from build123d import *

# Parameters (mm, degrees)
DODANIE_WYCI_GNI_CIE1_DEPTH = 6
WYTNIJ_WYCI_GNI_CIE2_DEPTH  = 4
WYTNIJ_WYCI_GNI_CIE3_DEPTH  = 2


with BuildPart() as part:
    # Szkic1 → Dodanie-wyciągnięcie1 (new body)
    with BuildSketch(Plane.XY):
        with BuildLine():
            Line((-16.5, 21.5), (16.5, 21.5))
            ThreePointArc((16.5, 21.5), (20.035533906, 20.035533906), (21.5, 16.5))
            Line((21.5, 16.5), (21.5, -16.5))
            ThreePointArc((21.5, -16.5), (20.035533906, -20.035533906), (16.5, -21.5))
            Line((16.5, -21.5), (-16.5, -21.5))
            ThreePointArc((-16.5, -21.5), (-20.035533906, -20.035533906), (-21.5, -16.5))
            Line((-21.5, -16.5), (-21.5, 16.5))
            ThreePointArc((-21.5, 16.5), (-20.035533906, 20.035533906), (-16.5, 21.5))
        make_face()
    extrude(amount=DODANIE_WYCI_GNI_CIE1_DEPTH)

    # Szkic2 → Wytnij-wyciągnięcie2 (cut)
    with BuildSketch(Plane.XY.offset(6)):
        with BuildLine():
            Line((-16.5, 1.360589702), (-16.5, -1.360589702))
            ThreePointArc((-16.5, -1.360589702), (-16.720373698, -2.828640251), (-17.362068966, -4.167282908))
            ThreePointArc((-17.362068966, -4.167282908), (-16.217514421, -16.217514421), (-4.167282908, -17.362068966))
            ThreePointArc((-4.167282908, -17.362068966), (-2.828640251, -16.720373698), (-1.360589702, -16.5))
            Line((-1.360589702, -16.5), (1.360589702, -16.5))
            ThreePointArc((1.360589702, -16.5), (2.828640251, -16.720373698), (4.167282908, -17.362068966))
            ThreePointArc((4.167282908, -17.362068966), (16.217514421, -16.217514421), (17.362068966, -4.167282908))
            ThreePointArc((17.362068966, -4.167282908), (16.720373698, -2.828640251), (16.5, -1.360589702))
            Line((16.5, -1.360589702), (16.5, 1.360589702))
            ThreePointArc((16.5, 1.360589702), (16.720373698, 2.828640251), (17.362068966, 4.167282908))
            ThreePointArc((17.362068966, 4.167282908), (16.217514421, 16.217514421), (4.167282908, 17.362068966))
            ThreePointArc((4.167282908, 17.362068966), (2.828640251, 16.720373698), (1.360589702, 16.5))
            Line((1.360589702, 16.5), (-1.360589702, 16.5))
            ThreePointArc((-1.360589702, 16.5), (-2.828640251, 16.720373698), (-4.167282908, 17.362068966))
            ThreePointArc((-4.167282908, 17.362068966), (-16.217514421, 16.217514421), (-17.362068966, 4.167282908))
            ThreePointArc((-17.362068966, 4.167282908), (-16.720373698, 2.828640251), (-16.5, 1.360589702))
        make_face()
    extrude(amount=-WYTNIJ_WYCI_GNI_CIE2_DEPTH, mode=Mode.SUBTRACT)

    # Szkic3 → Wytnij-wyciągnięcie3 (cut)
    with BuildSketch(Plane.XY.offset(2)):
        with BuildLine():
            Line((6.5, -5.5), (12.5, -5.5))
            ThreePointArc((12.5, -5.5), (13.207106781, -5.792893219), (13.5, -6.5))
            Line((13.5, -6.5), (13.5, -12.5))
            ThreePointArc((13.5, -12.5), (13.207106781, -13.207106781), (12.5, -13.5))
            Line((12.5, -13.5), (6.5, -13.5))
            ThreePointArc((6.5, -13.5), (5.792893219, -13.207106781), (5.5, -12.5))
            Line((5.5, -12.5), (5.5, -6.5))
            ThreePointArc((5.5, -6.5), (5.792893219, -5.792893219), (6.5, -5.5))
        make_face()
        with BuildLine():
            Line((6.5, 13.5), (12.5, 13.5))
            ThreePointArc((12.5, 13.5), (13.207106781, 13.207106781), (13.5, 12.5))
            Line((13.5, 12.5), (13.5, 6.5))
            ThreePointArc((13.5, 6.5), (13.207106781, 5.792893219), (12.5, 5.5))
            Line((12.5, 5.5), (6.5, 5.5))
            ThreePointArc((6.5, 5.5), (5.792893219, 5.792893219), (5.5, 6.5))
            Line((5.5, 6.5), (5.5, 12.5))
            ThreePointArc((5.5, 12.5), (5.792893219, 13.207106781), (6.5, 13.5))
        make_face()
        with BuildLine():
            Line((-12.5, -5.5), (-6.5, -5.5))
            ThreePointArc((-6.5, -5.5), (-5.792893219, -5.792893219), (-5.5, -6.5))
            Line((-5.5, -6.5), (-5.5, -12.5))
            ThreePointArc((-5.5, -12.5), (-5.792893219, -13.207106781), (-6.5, -13.5))
            Line((-6.5, -13.5), (-12.5, -13.5))
            ThreePointArc((-12.5, -13.5), (-13.207106781, -13.207106781), (-13.5, -12.5))
            Line((-13.5, -12.5), (-13.5, -6.5))
            ThreePointArc((-13.5, -6.5), (-13.207106781, -5.792893219), (-12.5, -5.5))
        make_face()
        with BuildLine():
            Line((-12.5, 13.5), (-6.5, 13.5))
            ThreePointArc((-6.5, 13.5), (-5.792893219, 13.207106781), (-5.5, 12.5))
            Line((-5.5, 12.5), (-5.5, 6.5))
            ThreePointArc((-5.5, 6.5), (-5.792893219, 5.792893219), (-6.5, 5.5))
            Line((-6.5, 5.5), (-12.5, 5.5))
            ThreePointArc((-12.5, 5.5), (-13.207106781, 5.792893219), (-13.5, 6.5))
            Line((-13.5, 6.5), (-13.5, 12.5))
            ThreePointArc((-13.5, 12.5), (-13.207106781, 13.207106781), (-12.5, 13.5))
        make_face()
    extrude(amount=-WYTNIJ_WYCI_GNI_CIE3_DEPTH, mode=Mode.SUBTRACT)


solid = part.part
Work out the finished part from the listing and answer in its coordinate system (mm). A direction names the side the tool comes from. Give positions to 0.01 mm unless a question says otherwise; leave off trailing zeros. Loops run counter-clockwise (first coordinate to the right, second up) from the corner with the lowest first, then second, coordinate; pieces in that order, holes last. Notation, with made-up numbers: (-3.75, 22) -> (50.25, 22) arc R21 cw to (50.25, 48) -> close; hole circle Ø4 at (69, 30.5). An arc over 180 degrees is marked (long way). Use a Markdown table: item, result. Add a question column.
1. Determine the mould class of faces 4 (the cylindrical face through (13.215, -13.199, 1.014)), 5 (the cylindrical face through (20, 20.07, 2.96)), 6 (the flat face through (0, 21.5, 3)) for opening direction X: released by +X, released by -X, zero draft, split by the parting line, or undercut.
2. Section B-B on y = 13 is taken. Determine the outline of the cut face in (x, z).
3. Section C-C on x = -11.5 is taken. Determine the outline of the cut face in (y, z), and give its area (3 significant figures).
4. Section A-A on z = 2.8 is taken. Determine the outline of the cut face in (x, y).
5. Flat-ended cylindrical pins translate along their axes: pin 1 Ø5 at (x, y) = (10.5, 9) entering from -Z; pin 2 Ø11.5 at (x, y) = (-1, 2.5) entering from +Z. Find the tip coordinate at first contact, or state that the pin passes through.
6. Section D-D on x = 3.5 is taken. Determine the outline of the cut face in (y, z), and give its area (3 significant figures).
7. For faces 1 (the flat face through (-13.5, 9, 1)), 2 (the cylindrical face through (2.809, -16.714, 4.028)), 3 (the flat face through (21.5, 0, 3)), determine the directions among +Z, -Z, +X, -X, +Y, -Y from which every point of the face is accessible in a straight line to the end or side of a thin tool.
8. Find the intervals of material crossed by probe 1 along Y at (x, z) = (-9, 0.5); probe 2 along Y at (x, z) = (17, 2.75); probe 3 along X at (y, z) = (9.5, 5.1), in increasing order.
Results below:
| question | item | result |
|---|---|---|
| 1 | face 4 | undercut |
| 1 | face 5 | released by +X |
| 1 | face 6 | zero draft |
| 2 | outline | (-21.5, 0) -> (-13.37, 0) -> (-13.37, 2) -> (-18.33, 2) -> (-18.33, 6) -> (-21.5, 6) -> close; (-5.63, 0) -> (5.63, 0) -> (5.63, 2) -> (-5.63, 2) -> close; (13.37, 0) -> (21.5, 0) -> (21.5, 6) -> (18.33, 6) -> (18.33, 2) -> (13.37, 2) -> close |
| 3 | outline | (-21.5, 0) -> (-13.5, 0) -> (-13.5, 2) -> (-18.79, 2) -> (-18.79, 6) -> (-21.5, 6) -> close; (-5.5, 0) -> (5.5, 0) -> (5.5, 2) -> (-5.5, 2) -> close; (13.5, 0) -> (21.5, 0) -> (21.5, 6) -> (18.79, 6) -> (18.79, 2) -> (13.5, 2) -> close |
| 3 | area | 75.7 mm^2 |
| 4 | outline | (-21.5, -16.5) arc R5 ccw to (-16.5, -21.5) -> (16.5, -21.5) arc R5 ccw to (21.5, -16.5) -> (21.5, 16.5) arc R5 ccw to (16.5, 21.5) -> (-16.5, 21.5) arc R5 ccw to (-21.5, 16.5) -> close; hole (-17.36, -4.17) arc R9.5 ccw to (-4.17, -17.36) arc R5 cw to (-1.36, -16.5) -> (1.36, -16.5) arc R5 cw to (4.17, -17.36) arc R9.5 ccw to (17.36, -4.17) arc R5 cw to (16.5, -1.36) -> (16.5, 1.36) arc R5 cw to (17.36, 4.17) arc R9.5 ccw to (4.17, 17.36) arc R5 cw to (1.36, 16.5) -> (-1.36, 16.5) arc R5 cw to (-4.17, 17.36) arc R9.5 ccw to (-17.36, 4.17) arc R5 cw to (-16.5, 1.36) -> (-16.5, -1.36) arc R5 cw to start |
| 5 | pin 1 | passes through |
| 5 | pin 2 | stops at z = 2 |
| 6 | outline | (-21.5, 0) -> (21.5, 0) -> (21.5, 6) -> (16.98, 6) -> (16.98, 2) -> (-16.98, 2) -> (-16.98, 6) -> (-21.5, 6) -> close |
| 6 | area | 122 mm^2 |
| 7 | face 1 | +Z, -Z |
| 7 | face 2 | +Z |
| 7 | face 3 | +Z, -Z, +X, +Y, -Y |
| 8 | probe 1 | y = -21.5 to -13.5, -5.5 to 5.5, 13.5 to 21.5 |
| 8 | probe 2 | y = -21.47 to -15.33, -3.54 to 3.54, 15.33 to 21.47 |
| 8 | probe 3 | x = -21.5 to -19, 19 to 21.5 |
